Read the model definition and answer for the solid it produces. Units are mm, in the model's axes. A direction names the side the tool comes from. Round coordinates to 2 decimals unless told otherwise and drop trailing zeros. Order: outer loops, then holes, each group sorted by start corner. A loop starts at its lowest first (then second) coordinate and runs counter-clockwise, first axis right, second up. Notation, with made-up numbers: (-5.5, 89) -> (36.5, 89) arc R13 ccw to (36.5, 111) -> close; hole circle Ø3 at (8, 53). An arc over 180 degrees is marked (long way). Use a Markdown table: item, result. Add a question column.
1. Section B-B, the plane x = 0 is taken. Give the vertices of the cut face in (y, z).
2. Section C-C, the plane y = 4 is taken. Give the vertices of the cut face in (x, z), then the cut area to 3 significant figures.
3. Section A-A, the plane y = 20 is taken. Give the vertices of the cut face in (x, z).
4. For faces 1 (the face through (4.713, 38.109, -12.325)), 2 (the face through (20, 32, -12)), 3 (the face through (0.1, 26.6, -12.3)), 4 (the face through (18.07, 24.7, -12.32)), determine the directions among +Z, -Z, +X, -X, +Y, -Y from which every point of the face is accessible in a straight line to the end or side of a thin tool.
5. The mould has two halves that part along Y. Classify faces 5 (the face through (-9.2, 9.4, -25)), 6 (the face through (0, -40, -12)), 7 (the face through (-10.51, -7.72, -12.32)), 8 (the face through (15.34, -12.92, -12.32)): +Y half, -Y half, draft (parallel to the pull), parting line (faces both ways), or undercut.
6. Consider L1, parallel to Y at x = 0, z = -15.75; L2, parallel to X at y = -22, z = -19.5; L3, parallel to X at y = 18.5, z = -3.75. Determine where each line is inside the solid, lowest interval first. Write a range as [from, to].
7. Given pin 1 (7.5 mm diameter, centred on y = 23.5, z = -8.5, fed in from +X), flat-ended and moving along its own axis, determine where the tip first touches the part or whether it passes through.
8. Section D-D, the plane z = -19 is taken. Give the number of separate pieces and of enclosed holes in the cut face, then the cut area to 3 significant figures.
```python
from build123d import *

# Parameters (mm, degrees)
SK_MAIN_EXTRUSION_R  = 3.4
MAIN_EXTRUSION_DEPTH = 25


with BuildPart() as part:
    # Sk Main Extrusion → Main Extrusion (new body)
    with BuildSketch(Plane.XY):
        with BuildLine():
            Line((16.671180212, -15.809923155), (19.506515107, -14.777945649))
            ThreePointArc((19.506515107, -14.777945649), (19.864364033, -14.503358511), (20, -14.073176184))
            Line((20, -14.073176184), (20, 14.073176184))
            ThreePointArc((20, 14.073176184), (19.864364033, 14.503358511), (19.506515107, 14.777945649))
            Line((19.506515107, 14.777945649), (16.671180212, 15.809923155))
            ThreePointArc((16.671180212, 15.809923155), (16.563886241, 15.824048675), (16.460675177, 15.791506351))
            Line((16.460675177, 15.791506351), (15.111296024, 15.012441934))
            Line((15.111296024, 15.012441934), (14.845251581, 14.281490834))
            Line((14.845251581, 14.281490834), (15.81984631, 11.603813821))
            ThreePointArc((15.81984631, 11.603813821), (15.786489799, 11.188925388), (15.450654467, 10.943039849))
            ThreePointArc((15.450654467, 10.943039849), (12.665882372, 11.066566987), (10.272684887, 12.495839661))
            Line((10.272684887, 12.495839661), (9.309262274, 13.459262274))
            ThreePointArc((9.309262274, 13.459262274), (6.6, 20), (9.309262274, 26.540737726))
            Line((9.309262274, 26.540737726), (10.272684887, 27.504160339))
            ThreePointArc((10.272684887, 27.504160339), (12.665882372, 28.933433013), (15.450654467, 29.056960151))
            ThreePointArc((15.450654467, 29.056960151), (15.786489799, 28.811074612), (15.81984631, 28.396186179))
            Line((15.81984631, 28.396186179), (14.845251581, 25.718509166))
            Line((14.845251581, 25.718509166), (15.111296024, 24.987558066))
            Line((15.111296024, 24.987558066), (16.460675177, 24.208493649))
            ThreePointArc((16.460675177, 24.208493649), (16.563886241, 24.175951325), (16.671180212, 24.190076845))
            Line((16.671180212, 24.190076845), (19.506515107, 25.222054351))
            ThreePointArc((19.506515107, 25.222054351), (19.864364033, 25.496641489), (20, 25.926823816))
            Line((20, 25.926823816), (20, 38.5))
            ThreePointArc((20, 38.5), (19.560660172, 39.560660172), (18.5, 40))
            Line((18.5, 40), (5.926823816, 40))
            ThreePointArc((5.926823816, 40), (5.496641489, 39.864364033), (5.222054351, 39.506515107))
            Line((5.222054351, 39.506515107), (4.190076845, 36.671180212))
            ThreePointArc((4.190076845, 36.671180212), (4.175951325, 36.563886241), (4.208493649, 36.460675177))
            Line((4.208493649, 36.460675177), (4.987558066, 35.111296024))
            Line((4.987558066, 35.111296024), (5.718509166, 34.845251581))
            Line((5.718509166, 34.845251581), (8.396186179, 35.81984631))
            ThreePointArc((8.396186179, 35.81984631), (8.811074612, 35.786489799), (9.056960151, 35.450654467))
            ThreePointArc((9.056960151, 35.450654467), (8.933433013, 32.665882372), (7.504160339, 30.272684887))
            Line((7.504160339, 30.272684887), (6.540737726, 29.309262274))
            ThreePointArc((6.540737726, 29.309262274), (0, 26.6), (-6.540737726, 29.309262274))
            Line((-6.540737726, 29.309262274), (-7.504160339, 30.272684887))
            ThreePointArc((-7.504160339, 30.272684887), (-8.933433013, 32.665882372), (-9.056960151, 35.450654467))
            ThreePointArc((-9.056960151, 35.450654467), (-8.811074612, 35.786489799), (-8.396186179, 35.81984631))
            Line((-8.396186179, 35.81984631), (-5.718509166, 34.845251581))
            Line((-5.718509166, 34.845251581), (-4.987558066, 35.111296024))
            Line((-4.987558066, 35.111296024), (-4.208493649, 36.460675177))
            ThreePointArc((-4.208493649, 36.460675177), (-4.175951325, 36.563886241), (-4.190076845, 36.671180212))
            Line((-4.190076845, 36.671180212), (-5.222054351, 39.506515107))
            ThreePointArc((-5.222054351, 39.506515107), (-5.496641489, 39.864364033), (-5.926823816, 40))
            Line((-5.926823816, 40), (-18.5, 40))
            ThreePointArc((-18.5, 40), (-19.560660172, 39.560660172), (-20, 38.5))
            Line((-20, 38.5), (-20, -38.5))
            ThreePointArc((-20, -38.5), (-19.560660172, -39.560660172), (-18.5, -40))
            Line((-18.5, -40), (18.5, -40))
            ThreePointArc((18.5, -40), (19.560660172, -39.560660172), (20, -38.5))
            Line((20, -38.5), (20, -25.926823816))
            ThreePointArc((20, -25.926823816), (19.864364033, -25.496641489), (19.506515107, -25.222054351))
            Line((19.506515107, -25.222054351), (16.671180212, -24.190076845))
            ThreePointArc((16.671180212, -24.190076845), (16.563886241, -24.175951325), (16.460675177, -24.208493649))
            Line((16.460675177, -24.208493649), (15.111296024, -24.987558066))
            Line((15.111296024, -24.987558066), (14.845251581, -25.718509166))
            Line((14.845251581, -25.718509166), (15.81984631, -28.396186179))
            ThreePointArc((15.81984631, -28.396186179), (15.786489799, -28.811074612), (15.450654467, -29.056960151))
            ThreePointArc((15.450654467, -29.056960151), (12.665882372, -28.933433013), (10.272684887, -27.504160339))
            Line((10.272684887, -27.504160339), (9.309262274, -26.540737726))
            ThreePointArc((9.309262274, -26.540737726), (6.6, -20), (9.309262274, -13.459262274))
            Line((9.309262274, -13.459262274), (10.272684887, -12.495839661))
            ThreePointArc((10.272684887, -12.495839661), (12.665882372, -11.066566987), (15.450654467, -10.943039849))
            ThreePointArc((15.450654467, -10.943039849), (15.786489799, -11.188925388), (15.81984631, -11.603813821))
            Line((15.81984631, -11.603813821), (14.845251581, -14.281490834))
            Line((14.845251581, -14.281490834), (15.111296024, -15.012441934))
            Line((15.111296024, -15.012441934), (16.460675177, -15.791506351))
            ThreePointArc((16.460675177, -15.791506351), (16.563886241, -15.824048675), (16.671180212, -15.809923155))
        make_face()
        with Locations((0, -20)):
            Circle(SK_MAIN_EXTRUSION_R, mode=Mode.SUBTRACT)
        with Locations((0, 20)):
            Circle(SK_MAIN_EXTRUSION_R, mode=Mode.SUBTRACT)
        with BuildLine():
            Line((-17.5, 37), (-17.5, 5.474873734))
            ThreePointArc((-17.5, 5.474873734), (-17.191341716, 5.012933968), (-16.646446609, 5.121320344))
            Line((-16.646446609, 5.121320344), (-5.236899672, 16.530867281))
            ThreePointArc((-5.236899672, 16.530867281), (-5.095239754, 16.81540054), (-5.153698917, 17.127825306))
            ThreePointArc((-5.153698917, 17.127825306), (-5.897648575, 19.833442852), (-5.307583096, 22.576734694))
            ThreePointArc((-5.307583096, 22.576734694), (-5.153883821, 24.359333373), (-6.230846881, 25.788120301))
            ThreePointArc((-6.230846881, 25.788120301), (-7.316529108, 26.555931161), (-8.308504679, 27.441495321))
            Line((-8.308504679, 27.441495321), (-9.444282589, 28.577273231))
            ThreePointArc((-9.444282589, 28.577273231), (-11.611987193, 32.430514315), (-11.464011904, 36.849169473))
            ThreePointArc((-11.464011904, 36.849169473), (-11.537349181, 37.295452819), (-11.940719521, 37.5))
            Line((-11.940719521, 37.5), (-17, 37.5))
            ThreePointArc((-17, 37.5), (-17.353553391, 37.353553391), (-17.5, 37))
        make_face(mode=Mode.SUBTRACT)
        with BuildLine():
            Line((-3.469132719, 14.763100328), (-17.353553391, 0.878679656))
            ThreePointArc((-17.353553391, 0.878679656), (-17.461939766, 0.716467982), (-17.5, 0.525126266))
            Line((-17.5, 0.525126266), (-17.5, -0.525126266))
            ThreePointArc((-17.5, -0.525126266), (-17.461939766, -0.716467982), (-17.353553391, -0.878679656))
            Line((-17.353553391, -0.878679656), (-3.469132719, -14.763100328))
            ThreePointArc((-3.469132719, -14.763100328), (-3.18459946, -14.904760246), (-2.872174694, -14.846301083))
            ThreePointArc((-2.872174694, -14.846301083), (-0.166557148, -14.102351425), (2.576734694, -14.692416904))
            ThreePointArc((2.576734694, -14.692416904), (4.359333373, -14.846116179), (5.788120301, -13.769153119))
            ThreePointArc((5.788120301, -13.769153119), (6.555931161, -12.683470892), (7.441495321, -11.691495321))
            Line((7.441495321, -11.691495321), (8.577273231, -10.555717411))
            ThreePointArc((8.577273231, -10.555717411), (12.430514315, -8.388012807), (16.849169473, -8.535988096))
            ThreePointArc((16.849169473, -8.535988096), (17.295452819, -8.462650819), (17.5, -8.059280479))
            Line((17.5, -8.059280479), (17.5, 8.059280479))
            ThreePointArc((17.5, 8.059280479), (17.295452819, 8.462650819), (16.849169473, 8.535988096))
            ThreePointArc((16.849169473, 8.535988096), (12.430514315, 8.388012807), (8.577273231, 10.555717411))
            Line((8.577273231, 10.555717411), (7.441495321, 11.691495321))
            ThreePointArc((7.441495321, 11.691495321), (6.555931161, 12.683470892), (5.788120301, 13.769153119))
            ThreePointArc((5.788120301, 13.769153119), (4.359333373, 14.846116179), (2.576734694, 14.692416904))
            ThreePointArc((2.576734694, 14.692416904), (-0.166557148, 14.102351425), (-2.872174694, 14.846301083))
            ThreePointArc((-2.872174694, 14.846301083), (-3.18459946, 14.904760246), (-3.469132719, 14.763100328))
        make_face(mode=Mode.SUBTRACT)
        with BuildLine():
            Line((-17.5, -5.474873734), (-17.5, -34.525126266))
            ThreePointArc((-17.5, -34.525126266), (-17.191341716, -34.987066032), (-16.646446609, -34.878679656))
            Line((-16.646446609, -34.878679656), (-5.236899672, -23.469132719))
            ThreePointArc((-5.236899672, -23.469132719), (-5.095239754, -23.18459946), (-5.153698917, -22.872174694))
            ThreePointArc((-5.153698917, -22.872174694), (-5.9, -20), (-5.153698917, -17.127825306))
            ThreePointArc((-5.153698917, -17.127825306), (-5.095239754, -16.81540054), (-5.236899672, -16.530867281))
            Line((-5.236899672, -16.530867281), (-16.646446609, -5.121320344))
            ThreePointArc((-16.646446609, -5.121320344), (-17.191341716, -5.012933968), (-17.5, -5.474873734))
        make_face(mode=Mode.SUBTRACT)
        with BuildLine():
            Line((-3.469132719, -25.236899672), (-14.878679656, -36.646446609))
            ThreePointArc((-14.878679656, -36.646446609), (-14.987066032, -37.191341716), (-14.525126266, -37.5))
            Line((-14.525126266, -37.5), (14.67102413, -37.5))
            ThreePointArc((14.67102413, -37.5), (17.499746132, -34.633125439), (14.59523355, -31.843063688))
            ThreePointArc((14.59523355, -31.843063688), (11.339316504, -31.263177929), (8.577273231, -29.444282589))
            Line((8.577273231, -29.444282589), (7.441495321, -28.308504679))
            ThreePointArc((7.441495321, -28.308504679), (6.555931161, -27.316529108), (5.788120301, -26.230846881))
            ThreePointArc((5.788120301, -26.230846881), (4.359333373, -25.153883821), (2.576734694, -25.307583096))
            ThreePointArc((2.576734694, -25.307583096), (-0.166557148, -25.897648575), (-2.872174694, -25.153698917))
            ThreePointArc((-2.872174694, -25.153698917), (-3.18459946, -25.095239754), (-3.469132719, -25.236899672))
        make_face(mode=Mode.SUBTRACT)
        with BuildLine():
            Line((17.5, 31.940719521), (17.5, 37.5))
            Line((17.5, 37.5), (11.940719521, 37.5))
            ThreePointArc((11.940719521, 37.5), (11.537349181, 37.295452819), (11.464011904, 36.849169473))
            ThreePointArc((11.464011904, 36.849169473), (11.844928721, 34.508523804), (11.540116235, 32.156756572))
            ThreePointArc((11.540116235, 32.156756572), (11.66791097, 31.66791097), (12.156756572, 31.540116235))
            ThreePointArc((12.156756572, 31.540116235), (14.508523804, 31.844928721), (16.849169473, 31.464011904))
            ThreePointArc((16.849169473, 31.464011904), (17.295452819, 31.537349181), (17.5, 31.940719521))
        make_face(mode=Mode.SUBTRACT)
    extrude(amount=-MAIN_EXTRUSION_DEPTH)


solid = part.part
```
Verdict:
| question | item | result |
|---|---|---|
| 1 | outline | (-40, -25) -> (-37.5, -25) -> (-37.5, 0) -> (-40, 0) -> close; (-25.9, -25) -> (-23.4, -25) -> (-23.4, 0) -> (-25.9, 0) -> close; (-16.6, -25) -> (-14.1, -25) -> (-14.1, 0) -> (-16.6, 0) -> close; (14.1, -25) -> (16.6, -25) -> (16.6, 0) -> (14.1, 0) -> close; (23.4, -25) -> (26.6, -25) -> (26.6, 0) -> (23.4, 0) -> close |
| 2 | outline | (-20, -25) -> (-14.23, -25) -> (-14.23, 0) -> (-20, 0) -> close; (17.5, -25) -> (20, -25) -> (20, 0) -> (17.5, 0) -> close |
| 2 | area | 207 mm2 |
| 3 | outline | (-20, -25) -> (-17.5, -25) -> (-17.5, 0) -> (-20, 0) -> close; (-5.9, -25) -> (-3.4, -25) -> (-3.4, 0) -> (-5.9, 0) -> close; (3.4, -25) -> (6.6, -25) -> (6.6, 0) -> (3.4, 0) -> close |
| 4 | face 1 | +Z, -Z, +Y |
| 4 | face 2 | +Z, -Z, +X, +Y, -Y |
| 4 | face 3 | +Z, -Z |
| 4 | face 4 | +Z, -Z, +X |
| 5 | face 5 | draft |
| 5 | face 6 | -Y half |
| 5 | face 7 | undercut |
| 5 | face 8 | undercut |
| 6 | L1 | y = [-40, -37.5], [-25.9, -23.4], [-16.6, -14.1], [14.1, 16.6], [23.4, 26.6] |
| 6 | L2 | x = [-20, -17.5], [-5.55, -2.75], [2.75, 6.82] |
| 6 | L3 | x = [-20, -17.5], [-5.71, -3.05], [3.05, 6.72] |
| 7 | pin 1 | stops at x = 20 |
| 8 | separate pieces | 1 |
| 8 | enclosed holes | 7 |
| 8 | area | 1,110 mm2 |
